Geometry: see drawing. Coordinates: mm, zero at the bounding-box minimum. Coordinates: 2 decimals unless noted, no trailing zeros. Order: outer loops, then holes, each group sorted by start corner. A loop starts at its lowest first (then second) coordinate and runs counter-clockwise, first axis right, second up.
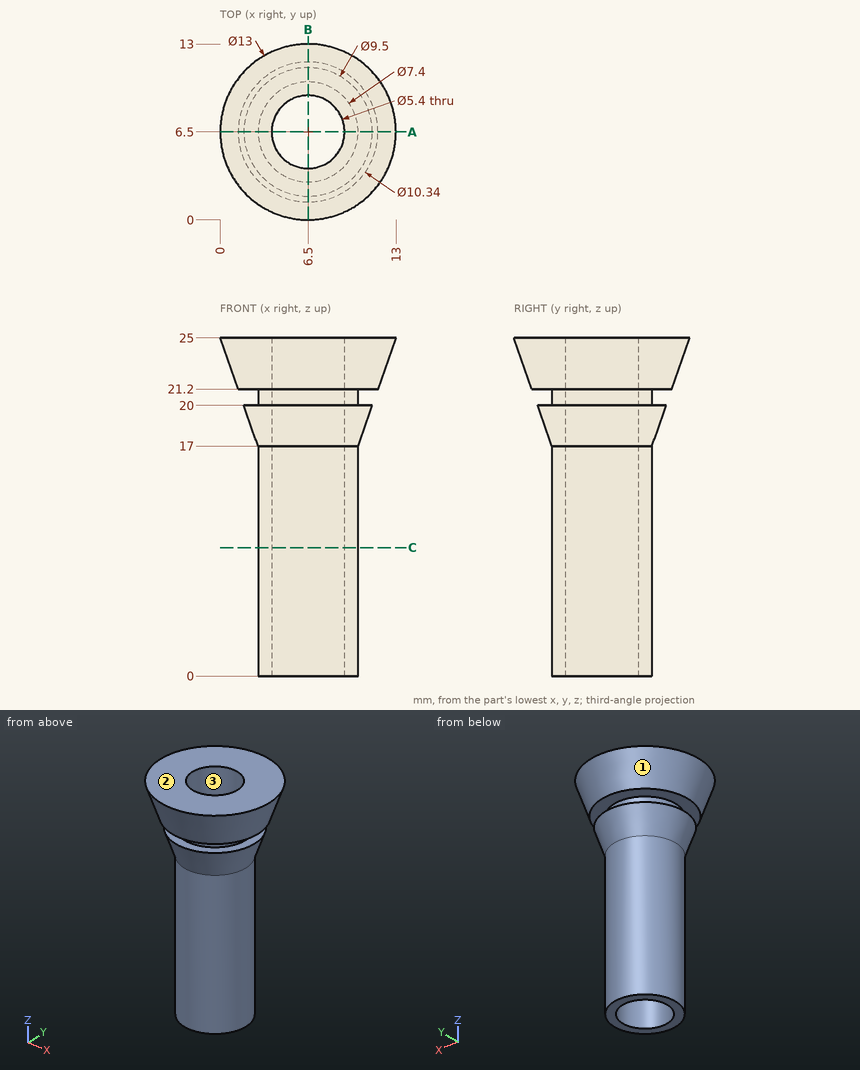
Item 1: Pin query (flat end, axial travel): pin 1 Ø3 at (x, z) = (3.5, 8.5) entering from +Y; pin 2 Ø5 at (x, y) = (8, 5.5) entering from +Z; pin 3 Ø5 at (y, z) = (4, 9) entering from +X; pin 4 Ø4 at (x, z) = (10, 17.5) entering from -Y. Return the tip coordinate at first contact, or that it passes through.
Response values:
pin 1: stops at y = 9.88
pin 2: stops at z = 25
pin 3: stops at x = 10.2
pin 4: stops at y = 2.65
Item 2: Cut plane A-A on y = 6.5. Return loops of the section in (x, z), then the cut area to 3 significant figures.
Response values:
outline: (0, 25) - (1.33, 21.2) - (2.8, 21.2) - (2.8, 20) - (1.75, 20) - (2.8, 17) - (2.8, 0) - (3.8, 0) - (3.8, 25) - close; (9.2, 0) - (10.2, 0) - (10.2, 17) - (11.25, 20) - (10.2, 20) - (10.2, 21.2) - (11.67, 21.2) - (13, 25) - (9.2, 25) - close
area: 69.4 mm2
Item 3: Ray query, probe 1 along Y at (x, z) = (6.5, 10.5); probe 2 along Y at (x, z) = (7.5, 18); probe 3 along X at (y, z) = (5, 10.75) (3 decimals). Return the intervals inside material, ascending.
Response values:
probe 1: y = 2.8 to 3.8, 9.2 to 10.2
probe 2: y = 2.58 to 3.99, 9.01 to 10.42
probe 3: x = 3.118 to 4.255, 8.745 to 9.882
Item 4: Cut plane C-C on z = 9.5. Return loops of the section in (x, y), then the cut area to 3 significant figures.
Response values:
outline: circle Ø7.4 at (6.5, 6.5); hole circle Ø5.4 at (6.5, 6.5)
area: 20.1 mm2
Item 5: Draft query along Y for the marked faces 1, 2 and 3. Return one class per face: pulls with the +Y half, pulls with the -Y half, needs draft (parallel to the pull), parting line crosses it, or undercut.
Response values:
face 1: parting line crosses it
face 2: needs draft
face 3: undercut
